Geometry: final body of the model. Coordinates: model frame, mm. A direction names the side the tool comes from. Round coordinates to 2 decimals unless told otherwise and drop trailing zeros. Loops run counter-clockwise (first coordinate to the right, second up) from the corner with the lowest first, then second, coordinate; pieces in that order, holes last. Notation, with made-up numbers: (18.25, 64.25) - (60.25, 64.25) arc R23 ccw to (60.25, 73.25) - close; hole circle Ø1 at (53.25, 14). An arc over 180 degrees is marked (long way). Answer in a Markdown table with one row per item. Add a question column.
from build123d import *

# Parameters (mm, degrees)
BOSS_EXTRUDE1_DEPTH = 3.2
BOSS_EXTRUDE2_START = 25.6
BOSS_EXTRUDE2_DEPTH = 25.6
SKETCH9_R           = 7
BOSS_EXTRUDE3_DEPTH = 25.6
BOSS_EXTRUDE4_DEPTH = 2
BOSS_EXTRUDE5_START = -46
BOSS_EXTRUDE5_DEPTH = 2
FILLET2_R           = 14
SKETCH12_R          = 1.75
CUT_EXTRUDE1_DEPTH  = 76.429503628
SKETCH15_R          = 3.5
CUT_EXTRUDE4_DEPTH  = 75.362423424
SKETCH16_R          = 1.75
CUT_EXTRUDE5_DEPTH  = 77.574734855
CUT_EXTRUDE6_DEPTH  = 3.7
FILLET3_R           = 5


with BuildPart() as part:
    # Sketch5 → Boss-Extrude1 (new body)
    with BuildSketch(Plane(origin=(0, 0, 0), x_dir=(1, 0, 0), z_dir=(0, 1, 0))):
        with BuildLine():
            Line((-62, 0), (62, 0))
            Line((62, 0), (62, 2.4))
            Line((62, 2.4), (51.5, 2.4))
            ThreePointArc((51.5, 2.4), (37.357864376, 8.257864376), (31.5, 22.4))
            Line((31.5, 22.4), (31.5, 34.5))
            Line((31.5, 34.5), (-31.5, 34.5))
            Line((-31.5, 34.5), (-31.5, 22.4))
            ThreePointArc((-31.5, 22.4), (-37.357864376, 8.257864376), (-51.5, 2.4))
            Line((-51.5, 2.4), (-62, 2.4))
            Line((-62, 2.4), (-62, 0))
        make_face()
    extrude(amount=-BOSS_EXTRUDE1_DEPTH)

    # Sketch8 → Boss-Extrude2 (add)
    with BuildSketch(Plane(origin=(0, 0, 0), x_dir=(1, 0, 0), z_dir=(0, 1, 0)).offset(BOSS_EXTRUDE2_START)):
        with BuildLine():
            Line((-35.807963803, 10), (35.807963803, 10))
            ThreePointArc((35.807963803, 10), (42.782202113, 4.4), (51.5, 2.4))
            Line((51.5, 2.4), (62, 2.4))
            Line((62, 2.4), (62, 0))
            Line((62, 0), (-62, 0))
            Line((-62, 0), (-62, 2.4))
            Line((-62, 2.4), (-51.5, 2.4))
            ThreePointArc((-51.5, 2.4), (-42.782202113, 4.4), (-35.807963803, 10))
        make_face()
    extrude(amount=-BOSS_EXTRUDE2_DEPTH)

    # Sketch9 → Boss-Extrude3 (add)
    with BuildSketch(Plane(origin=(0, 0, 0), x_dir=(1, 0, 0), z_dir=(0, 1, 0))):
        with Locations((-23, 10.6)):
            Circle(SKETCH9_R)
        with Locations((23, 10.6)):
            Circle(SKETCH9_R)
    extrude(amount=BOSS_EXTRUDE3_DEPTH)

    # Sketch10 → Boss-Extrude4 (add, symmetric)
    with BuildSketch(Plane(origin=(23, 0, 0), x_dir=(0, 0, -1), z_dir=(1, 0, 0))):
        Polygon((16.2, 16.6), (16.2, 0), (27.5, 0), align=None)
    extrude(amount=BOSS_EXTRUDE4_DEPTH, both=True)

    # Sketch10<4> → Boss-Extrude5 (add, symmetric)
    with BuildSketch(Plane(origin=(23, 0, 0), x_dir=(0, 0, -1), z_dir=(1, 0, 0)).offset(BOSS_EXTRUDE5_START)):
        Polygon((16.2, 16.6), (16.2, 0), (27.5, 0), align=None)
    extrude(amount=BOSS_EXTRUDE5_DEPTH, both=True)

    # Fillet2
    fillet2_edges = [part.edges().sort_by_distance(p)[0] for p in [
        (62, -3.2, -1.2),
        (62, 25.6, -1.2),
        (-62, -3.2, -1.2),
        (-62, 25.6, -1.2),
    ]]
    fillet(fillet2_edges, radius=FILLET2_R)

    # Sketch12 → Cut-Extrude1 (cut, through all)
    with BuildSketch(Plane.XY):
        with Locations((-47, 11.2)):
            Circle(SKETCH12_R)
        with Locations((47, 11.2)):
            Circle(SKETCH12_R)
    extrude(amount=-CUT_EXTRUDE1_DEPTH, mode=Mode.SUBTRACT)

    # Sketch15 → Cut-Extrude4 (cut, through all)
    with BuildSketch(Plane(origin=(0, 0, -2.4), x_dir=(-1, 0, 0), z_dir=(0, 0, -1))):
        with Locations(Location((-47, 11.2, 0), (0, 0, 180))):
            Circle(SKETCH15_R)
        with Locations(Location((47, 11.2, 0), (0, 0, 180))):
            Circle(SKETCH15_R)
    extrude(amount=CUT_EXTRUDE4_DEPTH, mode=Mode.SUBTRACT)

    # Sketch16 → Cut-Extrude5 (cut, through all)
    with BuildSketch(Plane(origin=(0, 25.6, 0), x_dir=(1, 0, 0), z_dir=(0, 1, 0))):
        with Locations(Location((-23, 10.6, 0), (0, 0, 270))):
            Circle(SKETCH16_R)
        with Locations(Location((23, 10.6, 0), (0, 0, 270))):
            Circle(SKETCH16_R)
    extrude(amount=-CUT_EXTRUDE5_DEPTH, mode=Mode.SUBTRACT)

    # Sketch17 → Cut-Extrude6 (cut)
    with BuildSketch(Plane(origin=(0, 25.6, 0), x_dir=(1, 0, 0), z_dir=(0, 1, 0))):
        with BuildLine():
            Line((-31.2, 21.2), (31.2, 21.2))
            ThreePointArc((31.2, 21.2), (41.8, 10.6), (31.2, 0))
            Line((31.2, 0), (-31.2, 0))
            ThreePointArc((-31.2, 0), (-41.8, 10.6), (-31.2, 21.2))
        make_face()
    extrude(amount=-CUT_EXTRUDE6_DEPTH, mode=Mode.SUBTRACT)

    # Fillet3
    fillet3_edges = [part.edges().sort_by_distance(p)[0] for p in [
        (16.02576169, 10.95, -10),
        (-29.97423831, 10.95, -10),
        (-16.02576169, 10.95, -10),
        (29.97423831, 10.95, -10),
    ]]
    fillet(fillet3_edges, radius=FILLET3_R)


solid = part.part
1) Material intervals for line 1 along Z through (x, y) = (-34.5, 10.25); line 2 along Y through (x, z) = (-12, -9.5); line 3 along X through (y, z) = (11.2, -2.95), sorted ascending. Write a range as from..to.
2) Section A-A, the plane y = 19. Return the cut outline in (x, z).
3) Section B-B, the plane x = 2. Return the cut outline in (y, z), and give its area (3 significant figures).
4) Section C-C, the plane y = 4.75. Return the cut outline in (x, z).
5) Reachability of faces 1 (the flat face through (21, 4, -20)), 2 (the flat face through (-25, 4, -20)), 3 (the cylindrical face through (31.39, 10.8, -10.84)), 4 (the cylindrical face through (48.617, 10.53, -1.183)), 5 (the cylindrical face through (-43.66, 10.15, -3.04)) from +Z, -Z, +X, -X, +Y, -Y: full face, straight path, thin tool, end or side. Return the list, or none.
6) Section D-D, the plane z = -31. Return the cut outline in (x, y), and give its area (3 significant figures).
7) Contact query for flat-ended pins moving along their axis: pin 1 Ø3 at (y, z) = (4.5, -20.5) entering from -X; pin 2 Ø5 at (y, z) = (16, -13) entering from -X; pin 3 Ø5 at (y, z) = (2.5, -7.5) entering from +X; pin 4 Ø2 at (x, y) = (47, 11.2) entering from -Z. Output: stop coordinate, or through.
8) Pull-direction query (Y, two-part tool) for faces 6 (the flat face through (-49, 12, -2.4)), 7 (the flat face through (45, 12, -2.4)), 8 (the cylindrical face through (-31.3, 10.8, -10.9)), 9 (the cylindrical face through (-57.8, 21.6, -1.4)); classes: pulls with the +Y half, pulls with the -Y half, needs draft (parallel to the pull), parting line crosses it, or undercut.
Evaluation:
| question | item | result |
|---|---|---|
| 1 | line 1 | z = -10..0 |
| 1 | line 2 | y = -3.2..21.9 |
| 1 | line 3 | x = -43.5..43.5 |
| 2 | outline | (-59.88, -2.4) - (-51.5, -2.4) arc R20 cw to (-35.81, -10) - (-34.16, -10) arc R5 cw to (-29.51, -13.17) arc R7 ccw to (-16.49, -13.17) arc R5 cw to (-11.84, -10) - (11.84, -10) arc R5 cw to (16.49, -13.17) arc R7 ccw to (29.51, -13.17) arc R5 cw to (34.16, -10) - (35.81, -10) arc R20 cw to (51.5, -2.4) - (59.88, -2.4) - (59.88, 0) - (-59.88, 0) - close; hole circle Ø3.5 at (-23, -10.6); hole circle Ø3.5 at (23, -10.6) |
| 3 | outline | (-3.2, -34.5) - (0, -34.5) - (0, -10) - (21.9, -10) - (21.9, 0) - (-3.2, 0) - close |
| 3 | area | 329 mm² |
| 4 | outline | (-60.63, -2.4) - (-51.5, -2.4) arc R20 cw to (-35.81, -10) - (-34.16, -10) arc R5 cw to (-29.51, -13.17) arc R7 ccw to (-25, -17.31) - (-25, -24.27) - (-21, -24.27) - (-21, -17.31) arc R7 ccw to (-16.49, -13.17) arc R5 cw to (-11.84, -10) - (11.84, -10) arc R5 cw to (16.49, -13.17) arc R7 ccw to (21, -17.31) - (21, -24.27) - (25, -24.27) - (25, -17.31) arc R7 ccw to (29.51, -13.17) arc R5 cw to (34.16, -10) - (35.81, -10) arc R20 cw to (51.5, -2.4) - (60.63, -2.4) - (60.63, 0) - (-60.63, 0) - close; hole circle Ø3.5 at (-23, -10.6); hole circle Ø3.5 at (23, -10.6) |
| 5 | face 1 | -Z, +Y |
| 5 | face 2 | -Z, -X, +Y |
| 5 | face 3 | -Z, +X, +Y |
| 5 | face 4 | +Z, -Z |
| 5 | face 5 | -Z |
| 6 | outline | (-31.5, -3.2) - (31.5, -3.2) - (31.5, 0) - (-31.5, 0) - close |
| 6 | area | 202 mm² |
| 7 | pin 1 | stops at x = -25 |
| 7 | pin 2 | stops at x = -31.98 |
| 7 | pin 3 | stops at x = 41.64 |
| 7 | pin 4 | passes through |
| 8 | face 6 | undercut |
| 8 | face 7 | undercut |
| 8 | face 8 | needs draft |
| 8 | face 9 | pulls with the +Y half |
